Verification items for the finished model (mm, model axes). Face numbers are marked on the shaded views. A direction names the side the tool comes from. Round coordinates to 2 decimals unless told otherwise and drop trailing zeros. Order: outer loops, then holes, each group sorted by start corner. A loop starts at its lowest first (then second) coordinate and runs counter-clockwise, first axis right, second up. Notation, with made-up numbers: (35, 28.5) -> (90, 28.5) arc R17 cw to (90, 35.5) -> close; hole circle Ø8 at (6.25, 31.25). An arc over 180 degrees is marked (long way). Write item = value, one per line. Start each with the question number.
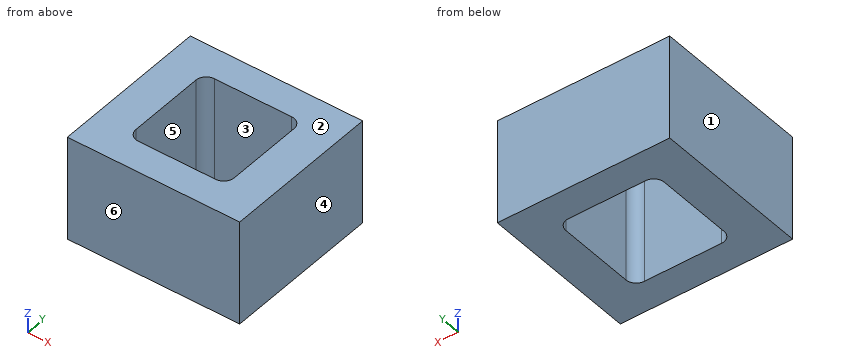
from build123d import *

# Parameters (mm, degrees)
F0_W     = 82.416646
F0_H     = 75.996064
F1_DEPTH = 50


with BuildPart() as f1:
    # F0 (on Top) → F1 (new body)
    with BuildSketch(Plane.XY):
        Rectangle(F0_W, F0_H)
        with BuildLine():
            ThreePointArc((23.5, -18.5), (22.035534, -22.035534), (18.5, -23.5))
            Line((18.5, -23.5), (-18.5, -23.5))
            ThreePointArc((-18.5, -23.5), (-22.035534, -22.035534), (-23.5, -18.5))
            Line((-23.5, -18.5), (-23.5, 18.5))
            ThreePointArc((-23.5, 18.5), (-22.035534, 22.035534), (-18.5, 23.5))
            Line((-18.5, 23.5), (18.5, 23.5))
            ThreePointArc((18.5, 23.5), (22.035534, 22.035534), (23.5, 18.5))
            Line((23.5, 18.5), (23.5, -18.5))
        make_face(mode=Mode.SUBTRACT)
    extrude(amount=F1_DEPTH)


solid = f1.part
(1) Draft check along X on the marked faces 1, 2, 3 and 4. Enter one of: +X half, -X half, draft (parallel to the pull), parting line (faces both ways), or undercut.
(2) Cross-section at A-A (y = -0.5). Enter the section's corners in (x, z).
(3) Cross-section at C-C (z = 34). Enter the section's corners in (x, y).
(4) Scan lines: line 1 along Y through (x, z) = (-9.5, 35); line 2 along X through (y, z) = (-7, 16.5). Record each from-to range of solid material in increasing order. Write a range as from..to.
(5) Cross-section at B-B (x = 3.5). Enter the section's corners in (y, z).
(6) Set-up check for the marked faces 5 and 6: record each of +Z, -Z, +X, -X, +Y, -Y from which the full face is reachable in a straight line by a thin tool's end or side.
Outcome:
q1.face_1 = -X half
q1.face_2 = draft
q1.face_3 = undercut
q1.face_4 = +X half
q2.outline = (-41.21, 0) -> (-23.5, 0) -> (-23.5, 50) -> (-41.21, 50) -> close; (23.5, 0) -> (41.21, 0) -> (41.21, 50) -> (23.5, 50) -> close
q3.outline = (-41.21, -38) -> (41.21, -38) -> (41.21, 38) -> (-41.21, 38) -> close; hole (-23.5, -18.5) arc R5 ccw to (-18.5, -23.5) -> (18.5, -23.5) arc R5 ccw to (23.5, -18.5) -> (23.5, 18.5) arc R5 ccw to (18.5, 23.5) -> (-18.5, 23.5) arc R5 ccw to (-23.5, 18.5) -> close
q4.line_1 = -38..-23.5, 23.5..38
q4.line_2 = -41.21..-23.5, 23.5..41.21
q5.outline = (-38, 0) -> (-23.5, 0) -> (-23.5, 50) -> (-38, 50) -> close; (23.5, 0) -> (38, 0) -> (38, 50) -> (23.5, 50) -> close
q6.face_5 = +Z, -Z
q6.face_6 = +Z, -Z, +X, -X, -Y
